Work out the finished part from the listing and answer in its coordinate system (mm). Face numbers are marked on the shaded views. A direction names the side the tool comes from. Round coordinates to 2 decimals unless told otherwise and drop trailing zeros. Loops run counter-clockwise (first coordinate to the right, second up) from the corner with the lowest first, then second, coordinate; pieces in that order, holes last. Notation, with made-up numbers: M 12,60.25 L 20,60.25 A16 cw 20,76.25 Z; hole C 18,63 d5. An arc over 180 degrees is marked long. One line per item, written item: value.
```python
from build123d import *
from build123d.topology import SkipClean

# Parameters (mm, degrees)
SKETCH2_R                        = 5.5
BOSS_EXTRUDE1_DEPTH              = 19
CUT_EXTRUDE1_DEPTH               = 35.190641995
CUT_EXTRUDE1_DEPTH_BACK          = 35.190641995
SKETCH3_W                        = 11
SKETCH3_H                        = 18
SKETCH4_W                        = 8.5
SKETCH4_H                        = 5.5
CUT_EXTRUDE4_DEPTH               = 19
SKETCH5_W                        = 19
SKETCH5_H                        = 18
SKETCH5_R                        = 8
BOSS_EXTRUDE4_DEPTH              = 20
F_3DSKETCH1_R                    = 8
BOSS_EXTRUDE5_DEPTH              = 18
BOSS_EXTRUDE8_DEPTH              = 10
BOSS_EXTRUDE19_REACH             = 53.078
SKETCH8_W                        = 18.6
SKETCH8_H                        = 7
SKETCH8_R                        = 2.1
BOSS_EXTRUDE19_DIRECTION_2_DEPTH = 14
SKETCH8_13_W                     = 2
SKETCH8_13_H                     = 2.5
SKETCH8_13_H_2                   = 0.5
SKETCH8_13_R                     = 2.1
CUT_EXTRUDE7_DEPTH               = 10
BOSS_EXTRUDE20_DEPTH             = 18
BOSS_EXTRUDE20_DEPTH_BACK        = 10
BOSS_EXTRUDE22_START             = 3
SKETCH11_W                       = 18.6
SKETCH11_H                       = 7
SKETCH11_R                       = 2.1
BOSS_EXTRUDE22_DEPTH             = 3
BOSS_EXTRUDE23_DEPTH             = 21
SKETCH12_W                       = 18
SKETCH12_H                       = 15.4
BOSS_EXTRUDE26_DEPTH             = 18
SKETCH13_W                       = 14
SKETCH13_H                       = 14
SKETCH13_W_2                     = 2
CUT_EXTRUDE8_DEPTH               = 15.4


with BuildPart() as part:
    # Sketch2 → Boss-Extrude1 (new body)
    with BuildSketch(Plane(origin=(0, 0, 0), x_dir=(0, 0, -1), z_dir=(1, 0, 0))):
        with BuildLine():
            Line((0, 0), (18, 0))
            Line((18, 0), (18, 13))
            ThreePointArc((18, 13), (9, 22), (0, 13))
            Line((0, 13), (0, 0))
        make_face()
        with Locations((9, 13)):
            Circle(SKETCH2_R, mode=Mode.SUBTRACT)
    extrude(amount=BOSS_EXTRUDE1_DEPTH)

    # Sketch3 → Cut-Extrude1 (cut, two sides: drawn at the far end of the back side and taken through both)
    with BuildSketch(Plane.XY.offset(-CUT_EXTRUDE1_DEPTH_BACK)):
        with Locations((9.5, 13)):
            Rectangle(SKETCH3_W, SKETCH3_H)
    extrude(amount=CUT_EXTRUDE1_DEPTH + CUT_EXTRUDE1_DEPTH_BACK, mode=Mode.SUBTRACT)

    # Sketch4 → Cut-Extrude4 (cut)
    with BuildSketch(Plane(origin=(0, 0, 0), x_dir=(1, 0, 0), z_dir=(0, 1, 0))):
        with Locations((9.45, 9.05)):
            Rectangle(SKETCH4_W, SKETCH4_H)
    extrude(amount=CUT_EXTRUDE4_DEPTH, mode=Mode.SUBTRACT)

    # Sketch5 → Boss-Extrude4 (add)
    with BuildSketch(Plane.XZ):
        with Locations((9.5, -9)):
            Rectangle(SKETCH5_W, SKETCH5_H)
        with Locations(Location((9.5, -9, 0), (0, 0, 270))):
            Circle(SKETCH5_R, mode=Mode.SUBTRACT)
    extrude(amount=BOSS_EXTRUDE4_DEPTH)

    # 3DSketch1 → Boss-Extrude5 (add)
    with BuildSketch(Plane(origin=(0, -20, 0), x_dir=(0.7259526839058267, 0, -0.687744647910783), z_dir=(0, 1, 0))):
        Polygon((0, 0), (12.379403662, 13.06714831), (26.172504657, 0), (13.793100994, -13.06714831), align=None)
        with Locations(Location((13.086252328, 0, 0), (0, 0, 226.548157699))):
            Circle(F_3DSKETCH1_R, mode=Mode.SUBTRACT)
    extrude(amount=-BOSS_EXTRUDE5_DEPTH)

    # Sketch7 → Boss-Extrude8 (add)
    with BuildSketch(Plane.ZY):
        Polygon((0, -23.8), (0, -14.8), (-2, -14.8), (-2, -22.8), (-7, -22.8), (-7, -24.8), (0, -24.8), align=None)
        Polygon((-16, -14.8), (-18, -14.8), (-18, -23.8), (-18, -24.8), (-11, -24.8), (-11, -22.8), (-16, -22.8), align=None)
    extrude(amount=BOSS_EXTRUDE8_DEPTH)

    # Boss-Extrude19: up to this face of the body (flat: up to its plane)
    boss_extrude19_end = Plane(part.part.faces().sort_by_distance((0, -10.449751669, -9))[0])
    # Sketch8 → Boss-Extrude19 (add, up to the picked face)
    with BuildSketch(Plane.ZY.offset(10), mode=Mode.PRIVATE) as boss_extrude19_sk1:
        with Locations((-9, -21.3)):
            Rectangle(SKETCH8_W, SKETCH8_H)
        with Locations(Location((-14, -21.6, 0), (0, 0, 162.247209838))):
            Circle(SKETCH8_R, mode=Mode.SUBTRACT)
        with Locations(Location((-4, -21.6, 0), (0, 0, 214.849904579))):
            Circle(SKETCH8_R, mode=Mode.SUBTRACT)
    boss_extrude19_tool1 = split(extrude(boss_extrude19_sk1.sketch, amount=-BOSS_EXTRUDE19_REACH, mode=Mode.PRIVATE), bisect_by=boss_extrude19_end, keep=Keep.BOTH, mode=Mode.PRIVATE)
    add(boss_extrude19_tool1.solids().sort_by(Axis((-10, -21.218894, -9), (1, 0, 0)))[0])

    # Sketch8 → Boss-Extrude19 direction 2 (add)
    with SkipClean():  # the faces are left unmerged after this step: merging them gives an invalid solid
        with BuildSketch(Plane.ZY.offset(10)):
            with Locations((-9, -21.3)):
                Rectangle(SKETCH8_W, SKETCH8_H)
            with Locations(Location((-14, -21.6, 0), (0, 0, 162.247209838))):
                Circle(SKETCH8_R, mode=Mode.SUBTRACT)
            with Locations(Location((-4, -21.6, 0), (0, 0, 214.849904579))):
                Circle(SKETCH8_R, mode=Mode.SUBTRACT)
        extrude(amount=BOSS_EXTRUDE19_DIRECTION_2_DEPTH)
    add(part.part.scale(1), mode=Mode.REPLACE)  # the faces are merged on a copy

    # Sketch8<13> → Cut-Extrude7 (cut)
    with SkipClean():  # the faces are left unmerged after this step: merging them gives an invalid solid
        with BuildSketch(Plane.ZY.offset(10)):
            with Locations((-17, -16.55)):
                Rectangle(SKETCH8_13_W, SKETCH8_13_H)
            with Locations((-17, -15.05)):
                Rectangle(SKETCH8_13_W, SKETCH8_13_H_2)
            with Locations((-1, -16.55)):
                Rectangle(SKETCH8_13_W, SKETCH8_13_H)
            with Locations((-1, -15.05)):
                Rectangle(SKETCH8_13_W, SKETCH8_13_H_2)
            with Locations(Location((-14, -21.6, 0), (0, 0, 180))):
                Circle(SKETCH8_13_R)
            with Locations(Location((-4, -21.6, 0), (0, 0, 180))):
                Circle(SKETCH8_13_R)
        extrude(amount=-CUT_EXTRUDE7_DEPTH, mode=Mode.SUBTRACT)
    add(part.part.scale(1), mode=Mode.REPLACE)  # the faces are merged on a copy

    # Sketch8<14> → Boss-Extrude20 (add, two sides: drawn at the far end of the back side and taken through both)
    with BuildSketch(Plane.ZY.offset(10).offset(-BOSS_EXTRUDE20_DEPTH_BACK)):
        Polygon((-11, -24.8), (-18, -24.8), (-18.3, -24.8), (-18.3, -17.8), (-20.485605357, -17.8), (-20.8, -17.8), (-20.8, -27.3), (-18, -27.3), (0, -27.3), (2.8, -27.3), (2.8, -17.8), (0.3, -17.8), (0.3, -24.8), (0, -24.8), (-9, -24.8), align=None)
    extrude(amount=BOSS_EXTRUDE20_DEPTH + BOSS_EXTRUDE20_DEPTH_BACK)

    # Sketch11 → Boss-Extrude22 (add)
    with SkipClean():  # the faces are left unmerged after this step: merging them gives an invalid solid
        with BuildSketch(Plane.ZY.offset(24).offset(BOSS_EXTRUDE22_START)):
            with Locations((-9, -21.3)):
                Rectangle(SKETCH11_W, SKETCH11_H)
            with Locations(Location((-14, -21.6, 0), (0, 0, 180))):
                Circle(SKETCH11_R, mode=Mode.SUBTRACT)
            with Locations(Location((-4, -21.6, 0), (0, 0, 180))):
                Circle(SKETCH11_R, mode=Mode.SUBTRACT)
        extrude(amount=-BOSS_EXTRUDE22_DEPTH)
    add(part.part.scale(1), mode=Mode.REPLACE)  # the faces are merged on a copy

    # Sketch8<15> → Boss-Extrude23 (add)
    with BuildSketch(Plane.ZY.offset(10)):
        Polygon((-11, -24.8), (-18, -24.8), (-18.3, -24.8), (-18.3, -17.8), (-20.485605357, -17.8), (-20.8, -17.8), (-20.8, -27.3), (-18, -27.3), (0, -27.3), (2.8, -27.3), (2.8, -17.8), (0.3, -17.8), (0.3, -24.8), (0, -24.8), (-9, -24.8), align=None)
    extrude(amount=BOSS_EXTRUDE23_DEPTH)

    # Sketch12 → Boss-Extrude26 (add)
    with BuildSketch(Plane.ZY):
        with Locations((-9, -10.1)):
            Rectangle(SKETCH12_W, SKETCH12_H)
    extrude(amount=BOSS_EXTRUDE26_DEPTH)

    # Sketch13 → Cut-Extrude8 (cut)
    with BuildSketch(Plane(origin=(0, -2.4, 0), x_dir=(1, 0, 0), z_dir=(0, 1, 0))):
        with Locations((-9, 9)):
            Rectangle(SKETCH13_W, SKETCH13_H)
        with Locations((-1, 9)):
            Rectangle(SKETCH13_W_2, SKETCH13_H)
    extrude(amount=-CUT_EXTRUDE8_DEPTH, mode=Mode.SUBTRACT)


solid = part.part
```
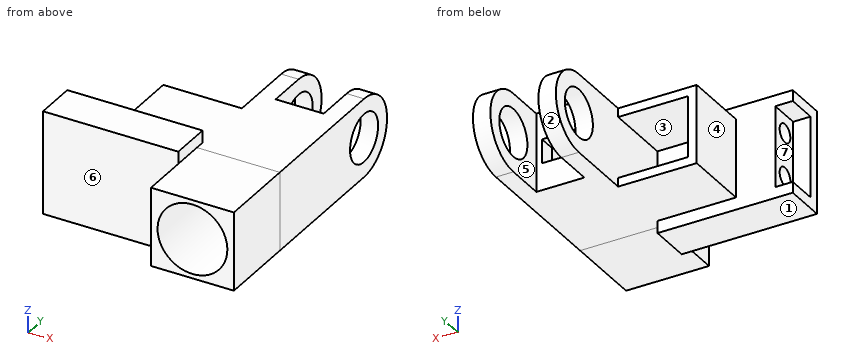
1) Find section B-B (y = -11.5). Give the vertices of the cut face in (x, z), then the cut area to 3 significant figures.
Check values:
outline: M -18,-18 L 19,-18 L 19,0 L -18,0 Z; hole M -16,-16 L 0,-16 L 0,-2 L -16,-2 Z; hole C 9.5,-9 d16
area: 241 mm2
2) For the marked faces 5, 6 and 7, determine the directions among +Z, -Z, +X, -X, +Y, -Y from which every point of the face is accessible in a straight line to the end or side of a thin tool.
Check values:
face 5: +Z, -Z, +Y
face 6: +Z, -Z, -X, -Y
face 7: -X, +Y
3) Each of these flat-tipped pins is pushed along its axis until it touches: pin 1 (5 mm diameter, centred on x = 1.5, y = 2, fed in from +Z); pin 2 (3 mm diameter, centred on x = -6, y = -12, fed in from -Z); pin 3 (0.7 mm diameter, centred on y = -23.5, z = -4.5, fed in from -X); pin 4 (6.5 mm diameter, centred on y = 13, z = -9, fed in from +X). Where does it stop, or does it pass through?
Check values:
pin 1: z = 0
pin 2: z = -18
pin 3: x = -27
pin 4: through
4) Find section A-A (x = -1.5). Give the vertices of the cut face in (y, z), then the cut area to 3 significant figures.
Check values:
outline: M -27.3,-20.8 L -17.8,-20.8 L -17.8,-18 L -2.4,-18 L -2.4,-16 L -17.8,-16 L -17.8,-2 L -2.4,-2 L -2.4,0 L -17.8,0 L -17.8,2.8 L -27.3,2.8 Z; hole C -21.6,-14 d4.2; hole C -21.6,-4 d4.2
area: 258 mm2
5) Find the intervals of material crossed by probe 1 along Z at (x, y) = (-26.05, -21.6); probe 2 along Y at (x, z) = (-13.75, -4); probe 3 along X at (y, z) = (13, -0.75), in increasing order. Write a range as from..to.
Check values:
probe 1: -20.8..-16.1, -11.9..-6.1, -1.9..2.8
probe 2: -27.3..-23.7, -19.5..-17.8
probe 3: 0..4, 15..19
6) Find section D-D (z = -9). Give the number of separate pieces and of enclosed holes in the cut face, then the cut area to 3 significant figures.
Check values:
separate pieces: 4
enclosed holes: 0
area: 509 mm2
7) Find section C-C (y = 9). Give the vertices of the cut face in (x, z), then the cut area to 3 significant figures.
Check values:
outline: M 0,-18 L 4,-18 L 4,-12.77 L 0,-12.77 Z; M 0,-5.23 L 4,-5.23 L 4,0 L 0,0 Z; M 15,-18 L 19,-18 L 19,-12.77 L 15,-12.77 Z; M 15,-5.23 L 19,-5.23 L 19,0 L 15,0 Z
area: 83.6 mm2
8) The mould has two halves that part along Z. Classify the marked faces 1, 2, 3 and 4: +Z half, -Z half, draft (parallel to the pull), parting line (faces both ways), or undercut.
Check values:
face 1: -Z half
face 2: parting line
face 3: undercut
face 4: draft
